The listing builds one solid part. Answer for the finished solid, in the listing's coordinates (mm). Face numbers are marked on the shaded views. Coordinates: 2 decimals unless noted, no trailing zeros. Write each loop counter-clockwise with the first axis right and the second up, starting at its lowest first coordinate (ties: lowest second). Pieces come first, ordered by that corner, then holes.
(1) The part is cut by section B-B on x = -35. Determine the outline of the cut face in (y, z), plus the area to 3 significant figures.
(2) Straight lines are drawn through the part: line 1 (X direction, y = 49, z = 125); line 2 (Z direction, x = 58, y = 37); line 3 (X direction, y = 27, z = -96). For each, find the intervals that lie inside material, in ascending order.
(3) The part is cut by section A-A on z = -120. Determine the outline of the cut face in (x, y).
(4) For a pull along Z with two mould halves and no side action, classify the marked faces 1, 2 and 3 as +Z half, -Z half, draft (parallel to the pull), parting line (faces both ways), or undercut.
(5) The part is cut by section D-D on z = -14.5. Determine the outline of the cut face in (x, y), plus the area to 4 significant figures.
(6) The part is cut by section C-C on y = 25. Give the number of separate pieces and of enclosed holes in the cut face, plus the area to 3 significant figures.
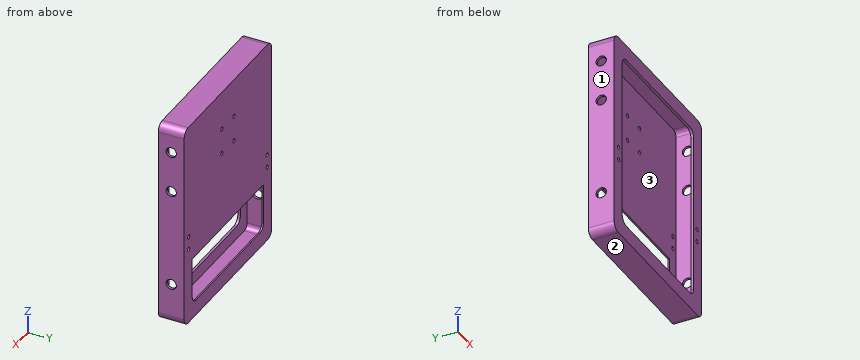
from build123d import *

# Parameters (mm, degrees)
BOSS_EXTRUDE1_DEPTH     = 50
SHELL1_T                = -5
SKETCH2_R               = 10
CUT_EXTRUDE1_DEPTH      = 325
BOSS_EXTRUDE2_DEPTH     = 3
CUT_EXTRUDE2_DEPTH      = 50
SKETCH6_R               = 4
CUT_EXTRUDE3_DEPTH      = 46
CUT_EXTRUDE3_DEPTH_BACK = 6
SKETCH7_W               = 265
SKETCH7_H               = 3
BOSS_EXTRUDE4_DEPTH     = 187
SKETCH8_R               = 4
CUT_EXTRUDE4_DEPTH      = 3
SKETCH7_2_W             = 265
SKETCH7_2_H             = 3
BOSS_EXTRUDE5_DEPTH     = 78


with BuildPart() as part:
    # Sketch1 → Boss-Extrude1 (new body)
    with BuildSketch(Plane(origin=(0, 0, 0), x_dir=(1, 0, 0), z_dir=(0, 1, 0))):
        with BuildLine():
            Line((-147.30160795, -200), (147.30160795, -200))
            ThreePointArc((147.30160795, -200), (158.048494032, -195.548494032), (162.5, -184.80160795))
            Line((162.5, -184.80160795), (162.5, 184.80160795))
            ThreePointArc((162.5, 184.80160795), (158.048494032, 195.548494032), (147.30160795, 200))
            Line((147.30160795, 200), (-147.30160795, 200))
            ThreePointArc((-147.30160795, 200), (-158.048494032, 195.548494032), (-162.5, 184.80160795))
            Line((-162.5, 184.80160795), (-162.5, -184.80160795))
            ThreePointArc((-162.5, -184.80160795), (-158.048494032, -195.548494032), (-147.30160795, -200))
        make_face()
    extrude(amount=BOSS_EXTRUDE1_DEPTH)

    # Shell1
    shell1_openings = [part.faces().sort_by_distance(p)[0] for p in [
        (0, 50, 0),
    ]]
    offset(amount=SHELL1_T, openings=shell1_openings, kind=Kind.INTERSECTION)

    # Sketch2 → Cut-Extrude1 (cut)
    with BuildSketch(Plane(origin=(162.5, 0, 0), x_dir=(0, 0, -1), z_dir=(1, 0, 0))):
        with Locations((-150, 25)):
            Circle(SKETCH2_R)
        with Locations((120, 25)):
            Circle(SKETCH2_R)
        with Locations((-70, 25)):
            Circle(SKETCH2_R)
    extrude(amount=-CUT_EXTRUDE1_DEPTH, mode=Mode.SUBTRACT)

    # Sketch3 → Boss-Extrude2 (add)
    with BuildSketch(Plane(origin=(0, 50, 0), x_dir=(1, 0, 0), z_dir=(0, 1, 0))):
        with BuildLine():
            Line((147.30160795, 195), (-147.30160795, 195))
            ThreePointArc((-147.30160795, 195), (-154.512960126, 192.012960126), (-157.5, 184.80160795))
            Line((-157.5, 184.80160795), (-157.5, -184.80160795))
            ThreePointArc((-157.5, -184.80160795), (-154.512960126, -192.012960126), (-147.30160795, -195))
            Line((-147.30160795, -195), (147.30160795, -195))
            ThreePointArc((147.30160795, -195), (154.512960126, -192.012960126), (157.5, -184.80160795))
            Line((157.5, -184.80160795), (157.5, 184.80160795))
            ThreePointArc((157.5, 184.80160795), (154.512960126, 192.012960126), (147.30160795, 195))
        make_face()
    extrude(amount=-BOSS_EXTRUDE2_DEPTH)

    # Sketch4 → Cut-Extrude2 (cut)
    with BuildSketch(Plane(origin=(0, 50, 0), x_dir=(1, 0, 0), z_dir=(0, 1, 0))):
        with BuildLine():
            Line((-117.30160795, -170), (117.30160795, -170))
            ThreePointArc((117.30160795, -170), (128.048494032, -165.548494032), (132.5, -154.80160795))
            Line((132.5, -154.80160795), (132.5, 154.80160795))
            ThreePointArc((132.5, 154.80160795), (128.048494032, 165.548494032), (117.30160795, 170))
            Line((117.30160795, 170), (-117.30160795, 170))
            ThreePointArc((-117.30160795, 170), (-128.048494032, 165.548494032), (-132.5, 154.80160795))
            Line((-132.5, 154.80160795), (-132.5, -154.80160795))
            ThreePointArc((-132.5, -154.80160795), (-128.048494032, -165.548494032), (-117.30160795, -170))
        make_face()
    extrude(amount=-CUT_EXTRUDE2_DEPTH, mode=Mode.SUBTRACT)

    # Sketch6 → Cut-Extrude3 (cut, two sides)
    with BuildSketch(Plane(origin=(0, 5, 0), x_dir=(1, 0, 0), z_dir=(0, 1, 0))) as cut_extrude3_sk:
        with Locations((-145.5, 50)):
            Circle(SKETCH6_R)
        with Locations((-145.5, 25)):
            Circle(SKETCH6_R)
        with Locations((145.5, 25)):
            Circle(SKETCH6_R)
        with Locations((145.5, 50)):
            Circle(SKETCH6_R)
    extrude(amount=CUT_EXTRUDE3_DEPTH, mode=Mode.SUBTRACT)
    extrude(cut_extrude3_sk.sketch, amount=-CUT_EXTRUDE3_DEPTH_BACK, mode=Mode.SUBTRACT)

    # Sketch7 → Boss-Extrude4 (add)
    with BuildSketch(Plane.XY):
        with Locations((0, 48.5)):
            Rectangle(SKETCH7_W, SKETCH7_H)
    extrude(amount=BOSS_EXTRUDE4_DEPTH)

    # Sketch8 → Cut-Extrude4 (cut)
    with BuildSketch(Plane(origin=(0, 50, 0), x_dir=(1, 0, 0), z_dir=(0, 1, 0))):
        with Locations((-22.5, -125)):
            Circle(SKETCH8_R)
        with Locations((-22.5, -75)):
            Circle(SKETCH8_R)
        with Locations((22.5, -125)):
            Circle(SKETCH8_R)
        with Locations((22.5, -75)):
            Circle(SKETCH8_R)
    extrude(amount=-CUT_EXTRUDE4_DEPTH, mode=Mode.SUBTRACT)

    # Sketch7<2> → Boss-Extrude5 (add)
    with BuildSketch(Plane.XY):
        with Locations((0, 48.5)):
            Rectangle(SKETCH7_2_W, SKETCH7_2_H)
    extrude(amount=-BOSS_EXTRUDE5_DEPTH)


solid = part.part
Model answer:
1. outline: (0, -200) - (50, -200) - (50, -170) - (47, -170) - (47, -195) - (5, -195) - (5, -170) - (0, -170) - close; (0, 170) - (5, 170) - (5, 195) - (47, 195) - (47, -78) - (50, -78) - (50, 200) - (0, 200) - close
1. area: 1,640 mm2
2. line 1: x = -162.5 to -26.5, -18.5 to 18.5, 26.5 to 162.5
2. line 2: z = -200 to -195, 195 to 200
2. line 3: x = -162.5 to -157.5, 157.5 to 162.5
3. outline: (-162.5, 0) - (-132.5, 0) - (-132.5, 5) - (-157.5, 5) - (-157.5, 15) - (-162.5, 15) - close; (-162.5, 35) - (-157.5, 35) - (-157.5, 47) - (-132.5, 47) - (-132.5, 50) - (-162.5, 50) - close; (132.5, 0) - (162.5, 0) - (162.5, 15) - (157.5, 15) - (157.5, 5) - (132.5, 5) - close; (132.5, 47) - (157.5, 47) - (157.5, 35) - (162.5, 35) - (162.5, 50) - (132.5, 50) - close
4. face 1: draft
4. face 2: -Z half
4. face 3: undercut
5. outline: (-162.5, 0) - (-132.5, 0) - (-132.5, 5) - (-157.5, 5) - (-157.5, 47) - (157.5, 47) - (157.5, 5) - (132.5, 5) - (132.5, 0) - (162.5, 0) - (162.5, 50) - (-162.5, 50) - close
5. area: 1,695 mm2
6. separate pieces: 6
6. enclosed holes: 0
6. area: 6,440 mm2
